```python
from build123d import *

# Parameters (mm, degrees)
F1_DEPTH = 300
F2_SIZE  = 13
F3_W     = 8
F3_H     = 300
F4_DEPTH = 3


with BuildPart() as f1:
    # F0 (on Front) → F1 (new body)
    with BuildSketch(Plane.XZ):
        Polygon((0, 226), (0, 0), (19, 19), (19, 207), align=None)
    extrude(amount=F1_DEPTH)

    # F2
    f2_edges = [f1.edges().sort_by_distance(p)[0] for p in [
        (19, -300, 113),
    ]]
    chamfer(f2_edges, length=F2_SIZE)

    # F3 (on face) → F4 (cut)
    with BuildSketch(Plane(origin=(0, 0, 0), x_dir=(-1, 0, 0), z_dir=(0, 1, 0))):
        with Locations((-15, 150)):
            Rectangle(F3_W, F3_H)
    extrude(amount=-F4_DEPTH, mode=Mode.SUBTRACT)


solid = f1.part
```
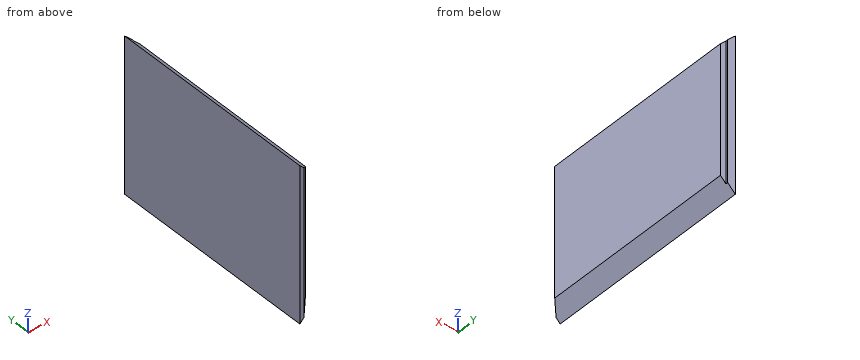
Geometry: final body of the model. Coordinates: model frame, mm. Coordinates: 2 decimals unless noted, no trailing zeros. Loops run counter-clockwise (first coordinate to the right, second up) from the corner with the lowest first, then second, coordinate; pieces in that order, holes last. Notation, with made-up numbers: (86, 32) -> (128, 32) arc R24 cw to (128, 62) -> close; hole circle Ø6 at (85.25, -37.75). An arc over 180 degrees is marked (long way). Use a Markdown table: item, result. Add a question column.
(1) Section query B-B, the plane x = 14.75. Return loops of the section in (y, z).
(2) Section query C-C, the plane y = -236.5. Return loops of the section in (x, z).
(3) Pin query (flat end, axial travel): pin 1 Ø6 at (x, y) = (6.5, -110) entering from +Z; pin 2 Ø3 at (y, z) = (-168, 41) entering from -X; pin 3 Ø0.9 at (y, z) = (-1, 134.5) entering from +X; pin 4 Ø3 at (x, y) = (3, -184) entering from -Z. Return the tip coordinate at first contact, or that it passes through.
(4) Section query A-A, the plane z = 74.5. Return loops of the section in (x, y).
(5) Line query: line 1 along Z through (x, y) = (4, -86.5); line 2 along Y through (x, z) = (17, 206); line 3 along Z through (x, y) = (18, -67). Output: solid intervals per line, ascending.
Answer:
| question | item | result |
|---|---|---|
| 1 | outline | (-291.25, 14.75) -> (-3, 14.75) -> (-3, 211.25) -> (-291.25, 211.25) -> close |
| 2 | outline | (0, 0) -> (19, 19) -> (19, 207) -> (0, 226) -> close |
| 3 | pin 1 | stops at z = 222.5 |
| 3 | pin 2 | stops at x = 0 |
| 3 | pin 3 | stops at x = 11 |
| 3 | pin 4 | stops at z = 1.5 |
| 4 | outline | (0, -300) -> (6, -300) -> (19, -287) -> (19, -3) -> (11, -3) -> (11, 0) -> (0, 0) -> close |
| 5 | line 1 | z = 4 to 222 |
| 5 | line 2 | y = -289 to -3 |
| 5 | line 3 | z = 18 to 208 |
